Source: CAD feature listing. Evaluate the final solid. Frame: model axes, mm. A direction names the side the tool comes from. Give positions to 0.01 mm unless a question says otherwise; leave off trailing zeros. Loops run counter-clockwise (first coordinate to the right, second up) from the corner with the lowest first, then second, coordinate; pieces in that order, holes last.
```python
from build123d import *

# Parameters (mm, degrees)
SKETCH_W   = 95.126476
SKETCH_H   = 31.708825
SKETCH_W_2 = 19.4
SKETCH_H_2 = 19.4
PAD_DEPTH  = 6
FILLET_R   = 2


with BuildPart() as part:
    # Sketch → Pad (new body)
    with BuildSketch(Plane.XY):
        with Locations((-0.29722, -0.938767)):
            Rectangle(SKETCH_W, SKETCH_H)
        with Locations((-32.5, -0.210358)):
            Rectangle(SKETCH_W_2, SKETCH_H_2, mode=Mode.SUBTRACT)
        with Locations((32.5, -0.210358)):
            Rectangle(SKETCH_W_2, SKETCH_H_2, mode=Mode.SUBTRACT)
    extrude(amount=PAD_DEPTH)

    # Fillet
    fillet_edges = [part.edges().sort_by_distance(p)[0] for p in [
        (47.266018, 14.915645, 3),
        (47.266018, -16.79318, 3),
        (-47.860458, 14.915645, 3),
        (-47.860458, -16.79318, 3),
    ]]
    fillet(fillet_edges, radius=FILLET_R)


solid = part.part
```
(1) Ray query, line 1 along X through (y, z) = (-1, 4.2); line 2 along Y through (x, z) = (30.5, 1.9). Return the intervals inside material, ascending.
A:
line 1: x = -47.86 to -42.2, -22.8 to 22.8, 42.2 to 47.27
line 2: y = -16.79 to -9.91, 9.49 to 14.92
(2) Reachability of faces 4 (the flat face through (-33, -9.91, 3)), 5 (the flat face through (47.266, -1, 3)) from +Z, -Z, +X, -X, +Y, -Y: full face, straight path, thin tool, end or side. Return the list, or none.
A:
face 4: +Z, -Z
face 5: +Z, -Z, +X, +Y, -Y
(3) Section A-A, the plane y = -2. Return the cut outline in (x, z).
A:
outline: (-47.86, 0) - (-42.2, 0) - (-42.2, 6) - (-47.86, 6) - close; (-22.8, 0) - (22.8, 0) - (22.8, 6) - (-22.8, 6) - close; (42.2, 0) - (47.27, 0) - (47.27, 6) - (42.2, 6) - close
(4) Section B-B, the plane x = 34. Return the cut outline in (y, z).
A:
outline: (-16.79, 0) - (-9.91, 0) - (-9.91, 6) - (-16.79, 6) - close; (9.49, 0) - (14.92, 0) - (14.92, 6) - (9.49, 6) - close
(5) Section C-C, the plane z = 1.65. Return the cut outline in (x, y), then the cut area to 3 significant figures.
A:
outline: (-47.86, -14.79) arc R2 ccw to (-45.86, -16.79) - (45.27, -16.79) arc R2 ccw to (47.27, -14.79) - (47.27, 12.92) arc R2 ccw to (45.27, 14.92) - (-45.86, 14.92) arc R2 ccw to (-47.86, 12.92) - close; hole (-42.2, -9.91) - (-22.8, -9.91) - (-22.8, 9.49) - (-42.2, 9.49) - close; hole (22.8, -9.91) - (42.2, -9.91) - (42.2, 9.49) - (22.8, 9.49) - close
area: 2,260 mm2
(6) Mould query, pull axis Y, two halves, no side actions, for faces 1 (the flat face through (-33, 9.49, 3)), 2 (the flat face through (-1, -1, 0)), 3 (the cylindrical face through (46.66, 14.35, 3.04)). Classes: pulls with the +Y half, pulls with the -Y half, needs draft (parallel to the pull), parting line crosses it, or undercut.
A:
face 1: undercut
face 2: needs draft
face 3: pulls with the +Y half
